```python
from build123d import *

# Parameters (mm, degrees)
SKETCH4_W                 = 10
SKETCH4_H                 = 57
BOSS_EXTRUDE3_DEPTH       = 2
SKETCH5_W                 = 10
SKETCH5_H                 = 2
BOSS_EXTRUDE4_DEPTH       = 2.05
SKETCH6_W                 = 10
SKETCH6_H                 = 2
BOSS_EXTRUDE5_DEPTH       = 15.9766
SKETCH7_W                 = 10
SKETCH7_H                 = 4
BOSS_EXTRUDE6_DEPTH       = 8.5
SKETCH8_W                 = 10
SKETCH8_H                 = 2
BOSS_EXTRUDE7_DEPTH       = 2.05
SKETCH9_W                 = 10
SKETCH9_H                 = 2
BOSS_EXTRUDE8_DEPTH       = 15.9766
SKETCH10_W                = 10
SKETCH10_H                = 2
BOSS_EXTRUDE9_DEPTH       = 8.5
F_6_CLEARANCE_HOLE1_D     = 3.6576
F_6_CLEARANCE_HOLE1_DEPTH = 7.62
F_6_CLEARANCE_HOLE1_TIP   = 1.0988539
FILLET2_R                 = 1
FILLET3_R                 = 2
SKETCH16_W                = 10
SKETCH16_H                = 2
BOSS_EXTRUDE10_DEPTH      = 2


with BuildPart() as part:
    # Sketch4 → Boss-Extrude3 (new body)
    with BuildSketch(Plane(origin=(0, 0, 0), x_dir=(1, 0, 0), z_dir=(0, 1, 0))):
        with Locations((11.706300269, -28.497829615)):
            Rectangle(SKETCH4_W, SKETCH4_H)
        with BuildLine():
            Line((13.706300269, -8.497829615), (13.706300269, -48.497829615))
            ThreePointArc((13.706300269, -48.497829615), (11.706300269, -50.497829615), (9.706300269, -48.497829615))
            Line((9.706300269, -48.497829615), (9.706300269, -8.497829615))
            ThreePointArc((9.706300269, -8.497829615), (11.706300269, -6.497829615), (13.706300269, -8.497829615))
        make_face(mode=Mode.SUBTRACT)
    extrude(amount=BOSS_EXTRUDE3_DEPTH)

    # Sketch5 → Boss-Extrude4 (add)
    with BuildSketch(Plane.XY.offset(56.997829615)):
        with Locations((11.706300269, 1)):
            Rectangle(SKETCH5_W, SKETCH5_H)
    extrude(amount=BOSS_EXTRUDE4_DEPTH)

    # Sketch6 → Boss-Extrude5 (add)
    with BuildSketch(Plane.XZ):
        with Locations((11.706300269, 58.047829615)):
            Rectangle(SKETCH6_W, SKETCH6_H)
    extrude(amount=BOSS_EXTRUDE5_DEPTH)

    # Sketch7 → Boss-Extrude6 (add)
    with BuildSketch(Plane.XY.offset(59.047829615)):
        with Locations((11.706300269, -15.9766)):
            Rectangle(SKETCH7_W, SKETCH7_H)
    extrude(amount=BOSS_EXTRUDE6_DEPTH)

    # Sketch8 → Boss-Extrude7 (add)
    with BuildSketch(Plane(origin=(0, 0, -0.002170385), x_dir=(-1, 0, 0), z_dir=(0, 0, -1))):
        with Locations((-11.706300269, 1)):
            Rectangle(SKETCH8_W, SKETCH8_H)
    extrude(amount=BOSS_EXTRUDE7_DEPTH)

    # Sketch9 → Boss-Extrude8 (add)
    with BuildSketch(Plane.XZ):
        with Locations((11.706300269, -1.052170385)):
            Rectangle(SKETCH9_W, SKETCH9_H)
    extrude(amount=BOSS_EXTRUDE8_DEPTH)

    # Sketch10 → Boss-Extrude9 (add)
    with BuildSketch(Plane(origin=(0, 0, -2.052170385), x_dir=(-1, 0, 0), z_dir=(0, 0, -1))):
        with Locations((-11.706300269, -14.9766)):
            Rectangle(SKETCH10_W, SKETCH10_H)
    extrude(amount=BOSS_EXTRUDE9_DEPTH)

    # #6 Clearance Hole1
    with Locations(Plane(origin=(0, -13.9766, 0), x_dir=(1, 0, 0), z_dir=(0, 1, 0))):
        with Locations((11.706300269, -63.297829615), (11.706300269, 6.302170385)):
            Hole(F_6_CLEARANCE_HOLE1_D / 2, depth=F_6_CLEARANCE_HOLE1_DEPTH)
            with Locations((0, 0, -(F_6_CLEARANCE_HOLE1_DEPTH + F_6_CLEARANCE_HOLE1_TIP / 2))):  # 118° drill point
                Cone(0, F_6_CLEARANCE_HOLE1_D / 2, F_6_CLEARANCE_HOLE1_TIP, mode=Mode.SUBTRACT)

    # Fillet2
    fillet2_edges = [part.edges().sort_by_distance(p)[0] for p in [
        (11.706300269, 2, 59.047829615),
        (11.706300269, 2, -2.052170385),
    ]]
    fillet(fillet2_edges, radius=FILLET2_R)

    # Fillet3
    fillet3_edges = [part.edges().sort_by_distance(p)[0] for p in [
        (16.706300269, -15.9766, 67.547829615),
        (6.706300269, -15.9766, 67.547829615),
        (16.706300269, -14.9766, -10.552170385),
        (6.706300269, -14.9766, -10.552170385),
    ]]
    fillet(fillet3_edges, radius=FILLET3_R)

    # Sketch16 → Boss-Extrude10 (add)
    with BuildSketch(Plane(origin=(0, 0, 59.047829615), x_dir=(-1, 0, 0), z_dir=(0, 0, -1))):
        with Locations((-11.706300269, -16.9766)):
            Rectangle(SKETCH16_W, SKETCH16_H)
    extrude(amount=BOSS_EXTRUDE10_DEPTH)


solid = part.part
```
Read the model definition and answer for the solid it produces. Units are mm, in the model's axes. A direction names the side the tool comes from. Give positions to 0.01 mm unless a question says otherwise; leave off trailing zeros. Write each loop counter-clockwise with the first axis right and the second up, starting at its lowest first coordinate (ties: lowest second). Pieces come first, ordered by that corner, then holes. Notation, with made-up numbers: M 29,46.5 L 72,46.5 A27 cw 72,84.5 Z; hole C -35,-12 d3. An arc over 180 degrees is marked long. Put each result on its own line as item: value. Start each with the question number.
1. For a pull along X with two mould halves and no side action, classify faces 1 (the cylindrical face through (12.103, -14.991, -4.517)), 2 (the flat face through (12, -6, -2.052)), 3 (the cylindrical face through (16.136, -14.963, -9.951)) as released by +X, released by -X, zero draft, split by the parting line, or undercut.
2. Which of the six approach directions +Z, -Z, +X, -X, +Y, -Y give full straight-line access (tool end or side, diameter ignored) to faces 4 (the flat face through (9.55, 0, 28.9)), 5 (the flat face through (12, -13.977, -4)), 6 (the flat face through (12, -6, 59.048)), 7 (the cylindrical face through (11.75, 0.986, 50.497)), 8 (the flat face through (9.55, 2, 28.91))?
3. The part is cut by section B-B, the plane y = -11. Give the vertices of the cut face in (x, z).
4. The part is cut by section C-C, the plane x = 11. Give the vertices of the cut face in (y, z), and give its area (3 significant figures).
5. The part is cut by section A-A, the plane z = 17.5. Give the vertices of the cut face in (x, y), and give its area (3 significant figures).
6. Each of these flat-tipped pins is pushed along its axis until it touches: pin 1 Ø3 at (x, z) = (11.71, -6.3) entering from -Y; pin 2 Ø5 at (x, y) = (10.5, -4.5) entering from +Z; pin 3 Ø4 at (x, z) = (14, 62.5) entering from +Y; pin 4 Ø3 at (x, y) = (10, -12) entering from -Z. Where does it stop, or does it pass through?
7. The part is cut by section D-D, the plane x = 15.75. Give the vertices of the cut face in (y, z), and give its area (3 significant figures).
8. Consider line 1 along Z through (x, y) = (11.75, -14.25); line 2 along Z through (x, y) = (11.25, -12); line 3 along Y through (x, z) = (8.75, 55.5). Determine where each line is inside the solid, lowest interval first.
Final values:
1. face 1: undercut
1. face 2: zero draft
1. face 3: released by +X
2. face 4: +X, -X, -Y
2. face 5: -Z, +X, -X, +Y
2. face 6: +Z, +X, -X, +Y
2. face 7: +Y, -Y
2. face 8: +Z, -Z, +X, -X, +Y
3. outline: M 6.71,-2.05 L 16.71,-2.05 L 16.71,-0.05 L 6.71,-0.05 Z; M 6.71,57.05 L 16.71,57.05 L 16.71,59.05 L 6.71,59.05 Z
4. outline: M -17.98,57.05 L 0,57.05 L 0,50.37 L 2,50.37 L 2,58.05 A1 ccw 1,59.05 L -13.98,59.05 L -13.98,61.61 L -17.98,61.61 Z; M -17.98,64.98 L -13.98,64.98 L -13.98,67.55 L -17.98,67.55 Z; M -15.98,-10.55 L -13.98,-10.55 L -13.98,-7.99 L -15.98,-7.99 Z; M -15.98,-4.62 L -13.98,-4.62 L -13.98,-2.05 L 1,-2.05 A1 ccw 2,-1.05 L 2,6.63 L 0,6.63 L 0,-0.05 L -15.98,-0.05 Z
4. area: 133 mm²
5. outline: M 6.71,0 L 9.71,0 L 9.71,2 L 6.71,2 Z; M 13.71,0 L 16.71,0 L 16.71,2 L 13.71,2 Z
5. area: 12.0 mm²
6. pin 1: passes through
6. pin 2: stops at z = 59.05
6. pin 3: stops at y = -13.98
6. pin 4: stops at z = -2.05
7. outline: M -17.98,57.05 L 0,57.05 L 0,-0.05 L -15.98,-0.05 L -15.98,-10.26 L -13.98,-10.26 L -13.98,-2.05 L 1,-2.05 A1 ccw 2,-1.05 L 2,58.05 A1 ccw 1,59.05 L -13.98,59.05 L -13.98,67.25 L -17.98,67.25 Z
7. area: 239 mm²
8. line 1: z = -10.55 to -8.13, -4.47 to -0.05, 57.05 to 61.47, 65.13 to 67.55
8. line 2: z = -2.05 to -0.05, 57.05 to 59.05
8. line 3: y = 0 to 2
